Part model, mm, in its own coordinate system. A direction names the side the tool comes from. Give positions to 0.01 mm unless a question says otherwise; leave off trailing zeros. Write each loop counter-clockwise with the first axis right and the second up, starting at its lowest first coordinate (ties: lowest second). Pieces come first, ordered by that corner, then holes.
Autodesk Fusion 360 part; units mm, degrees
sketch "Sketch1" plane through (0, 0, 0) normal (0, 0, 1) x (1, 0, 0)
  circle A0 centre (-28, 0) radius 5
  circle A1 centre (0, 28) radius 5
  circle A2 centre (0, -28) radius 5
  line L0 (-0.0776, 15.9998) -> (36.6607, 15.9998)
  line L1 (-0.0776, -15.9998) -> (36.5825, -16.1777)
  arc A3 (36.6607, 15.9998) -> (36.5825, -16.1777) centre (0, 0) ccw
  arc A4 (0.0776, 15.9998) -> (-0.0776, -15.9998) centre (0, 0) ccw
  dimension "d1" = 80
  dimension "d3" = 28
  dimension "d4" = 10
  dimension "d5" = 28
  dimension "d6" = 28
  dimension "d7" = 10
  dimension "d8" = 10
extrude "Extrude1" add sketch "Sketch1" along normal blind 5
1) Mould opens along Y. For faces 1 (the cylindrical face through (-39.974, -1.43, 2.465)), 2 (the flat face through (-19, 1, 0)), 3 (the cylindrical face through (-33, 0, 2)), 4 (the cylindrical face through (-16, 0, 2)) say: +Y half, -Y half, draft (parallel to the pull), parting line (faces both ways), or undercut.
Check result:
face 1: parting line
face 2: draft
face 3: undercut
face 4: undercut
2) Saw through at D-D (y = 17.5). Write the cut outline in (x, z).
Check result:
outline: (-35.97, 0) - (35.97, 0) - (35.97, 5) - (-35.97, 5) - close
3) Flat gauge pins, fed straight in: P1, Ø1.5, axis at x = -1, z = 4, coming from the +Y side; P2, Ø3, axis at y = -9, z = 0.5, coming from the +X side; P3, Ø2, axis at x = -32, z = 4, coming from the +Y side. Where does each tip first touch, or does it go through?
Check result:
P1: stops at y = 40
P2: stops at x = -12.07
P3: stops at y = 25.28
4) Saw through at B-B (y = 0). Write the cut outline in (x, z), and give its area (3 significant figures).
Check result:
outline: (-40, 0) - (-33, 0) - (-33, 5) - (-40, 5) - close; (-23, 0) - (-16, 0) - (-16, 5) - (-23, 5) - close
area: 70.0 mm2
5) Drill centre lines: L1, parallel to Y at x = 0, z = 2.5; L2, parallel to X at y = 1.5, z = 3.5; L3, parallel to Y at x = 3.5, z = 0.45. Where is each one in solid material? Low to high.
Check result:
L1: y = -40 to -33, -23 to -16, 16 to 23, 33 to 40
L2: x = -39.97 to -32.77, -23.23 to -15.93
L3: y = -39.85 to -31.57, -24.43 to -16.02, 16 to 24.43, 31.57 to 39.85
6) Saw through at A-A (z = 3.55). Write the cut outline in (x, y), and give its area (3 significant figures).
Check result:
outline: (-0.08, -16) arc R16 cw to (-0.08, 16) - (36.66, 16) arc R40 ccw (long way) to (36.58, -16.18) - close; hole circle Ø10 at (-28, 0); hole circle Ø10 at (0, -28); hole circle Ø10 at (0, 28)
area: 3,140 mm2
7) Saw through at C-C (x = 20). Write the cut outline in (y, z).
Check result:
outline: (-34.64, 0) - (-16.1, 0) - (-16.1, 5) - (-34.64, 5) - close; (16, 0) - (34.64, 0) - (34.64, 5) - (16, 5) - close
8) 3-axis set-ups, long thin cutter, end or side, ignore diameter. For faces 5 (the flat face through (-19, 1, 5)), 6 (the flat face through (18, 16, 2)): which of +Z, -Z, +X, -X, +Y, -Y reach the whole face in a straight line?
Check result:
face 5: +Z, +X, -X, +Y, -Y
face 6: +Z, -Z, +X
